Can you work these out from the model? Positions are in its coordinate system, mm. A direction names the side the tool comes from. Round coordinates to 2 decimals unless told otherwise and drop trailing zeros. Loops run counter-clockwise (first coordinate to the right, second up) from the corner with the lowest first, then second, coordinate; pieces in that order, holes last. Notation, with made-up numbers: M 47.25,-5.5 L 65.25,-5.5 A16 ccw 65.25,12.5 Z; hole C -35,79.25 d5. An arc over 180 degrees is marked long. Answer as CSV lines item,"result".
from build123d import *

# Parameters (mm, degrees)
SKETCH_1_R          = 1.6
EXTRUDE_1_DEPTH     = 3
SKETCH_2_W          = 20
SKETCH_2_H          = 2
EXTRUDE_2_DEPTH     = 13
CUT_EXTRUDE_1_DEPTH = 20


with BuildPart() as part:
    # 草图1 → 凸台-拉伸1 (new body)
    with BuildSketch(Plane.XY):
        with BuildLine():
            Line((0, 0), (20, 0))
            Line((20, 0), (20, 17))
            ThreePointArc((20, 17), (19.121320344, 19.121320344), (17, 20))
            Line((17, 20), (0, 20))
            Line((0, 20), (0, 0))
        make_face()
        with Locations((17, 17)):
            Circle(SKETCH_1_R, mode=Mode.SUBTRACT)
        with Locations((17, 5)):
            Circle(SKETCH_1_R, mode=Mode.SUBTRACT)
    extrude(amount=EXTRUDE_1_DEPTH)

    # 草图2 → 凸台-拉伸2 (add)
    with BuildSketch(Plane.XY.offset(3)):
        with Locations((10, 1)):
            Rectangle(SKETCH_2_W, SKETCH_2_H)
    extrude(amount=-EXTRUDE_2_DEPTH)

    # 草图3 → 切除-拉伸1 (cut)
    with BuildSketch(Plane.XY.offset(3)):
        Polygon((0, 2), (15, 20), (0, 20), align=None)
    extrude(amount=-CUT_EXTRUDE_1_DEPTH, mode=Mode.SUBTRACT)


solid = part.part
Item 1: Will these pins go through, and if not, where does the flat tip stop? pin 1 (4 mm diameter, centred on x = 8.5, y = 14.5, fed in from -Z); pin 2 (1.5 mm diameter, centred on x = 11, z = -4, fed in from +Y).
Output:
pin 1,"stops at z = 0"
pin 2,"stops at y = 2"
Item 2: If I drill on line 1 along Y through (x, z) = (17, 2); line 2 along Y through (x, z) = (13, -1.75); line 3 along Z through (x, y) = (12, 10.5), over which ranges is the centre line in solid material (lowest first)? Write a range as from..to.
Output:
line 1,"y = 0..3.4, 6.6..15.4, 18.6..20"
line 2,"y = 0..2"
line 3,"z = 0..3"
Item 3: On a 3-axis mill with a long thin cutter (end or side, diameter ignored), from which of +Z, -Z, +X, -X, +Y, -Y can I reach the whole of each face in a straight line? I mean faces 4 (the face through (12, 9, 0)), 5 (the face through (10, 0, -3)). Say none if no direction works.
Output:
face 4,"-Z, +X, -X, +Y"
face 5,"+Z, -Z, +X, -X, -Y"
Item 4: If we section it at D-D on z = -7: Write out the boundary of the cut face in (x, y), then the cut area to 3 significant figures.
Output:
outline,"M 0,0 L 20,0 L 20,2 L 0,2 Z"
area,"40.0 mm2"
Item 5: We'd pull the mould along X, two halves only. Please class faces 1 (the face through (15.4, 5.07, 1.48)), 2 (the face through (16, 20, 1)), 3 (the face through (20, 6.6, 0.4)): released by +X, released by -X, zero draft, split by the parting line, or undercut.
Output:
face 1,"undercut"
face 2,"zero draft"
face 3,"released by +X"
Item 6: If we section it at C-C on y = 6.25: Write out the boundary of the cut face in (x, z), then the cut area to 3 significant figures.
Output:
outline,"M 3.54,0 L 16,0 L 16,3 L 3.54,3 Z; M 18,0 L 20,0 L 20,3 L 18,3 Z"
area,"43.4 mm2"
Item 7: If we section it at A-A on z = 1: Write out the boundary of the cut face in (x, y).
Output:
outline,"M 0,0 L 20,0 L 20,17 A3 ccw 17,20 L 15,20 L 0,2 Z; hole C 17,5 d3.2; hole C 17,17 d3.2"
Item 8: If we section it at B-B on x = 10.5: Write out the boundary of the cut face in (y, z).
Output:
outline,"M 0,-10 L 2,-10 L 2,0 L 14.6,0 L 14.6,3 L 0,3 Z"
